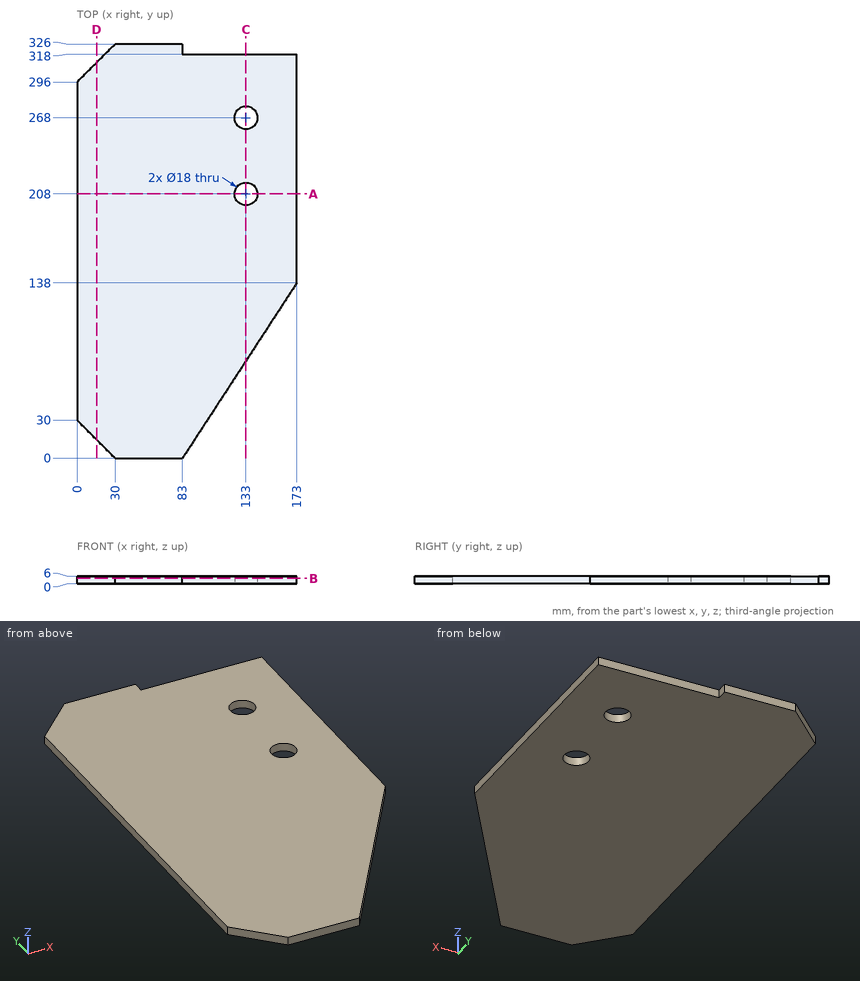
Source: three-view drawing plus pictorial views. Frame: mm from the lowest corner of the part. Coordinates: 2 decimals unless noted, no trailing zeros. Write each loop counter-clockwise with the first axis right and the second up, starting at its lowest first coordinate (ties: lowest second). Pieces come first, ordered by that corner, then holes. Notation, with made-up numbers: (69.5, 43) -> (105.5, 43) arc R25 cw to (105.5, 76) -> close; hole circle Ø1 at (34, 20). An arc over 180 degrees is marked (long way). Answer as a JSON object with one key per item and string values.
1. Section A-A on y = 208. Return the cut outline in (x, z).
Result set:
{"outline": "(0, 0) -> (124, 0) -> (124, 6) -> (0, 6) -> close; (142, 0) -> (173, 0) -> (173, 6) -> (142, 6) -> close"}
2. Section B-B on z = 4.2. Return the cut outline in (x, y).
Result set:
{"outline": "(0, 30) -> (30, 0) -> (83, 0) -> (173, 138) -> (173, 318) -> (83, 318) -> (83, 326) -> (30, 326) -> (0, 296) -> close; hole circle Ø18 at (133, 208); hole circle Ø18 at (133, 268)"}
3. First-contact query: P1, Ø16, axis at x = 133, y = 208, coming from the +Z side; P2, Ø1.8, axis at x = 122, z = 2.5, coming from the +Y side. Flat tips, straight axial feed; report the tip coordinate or a pass-through.
Result set:
{"P1": "passes through", "P2": "stops at y = 318"}
4. Material intervals for line 1 (Y direction, x = 133, z = 2.25); line 2 (X direction, y = 208, z = 2); line 3 (Y direction, x = 138, z = 2), sorted ascending. Write a range as from..to.
Result set:
{"line 1": "y = 76.67..199, 217..259, 277..318", "line 2": "x = 0..124, 142..173", "line 3": "y = 84.33..200.52, 215.48..260.52, 275.48..318"}
5. Section C-C on x = 133. Return the cut outline in (y, z), then the cut area to 3 significant figures.
Result set:
{"outline": "(76.67, 0) -> (199, 0) -> (199, 6) -> (76.67, 6) -> close; (217, 0) -> (259, 0) -> (259, 6) -> (217, 6) -> close; (277, 0) -> (318, 0) -> (318, 6) -> (277, 6) -> close", "area": "1,230 mm2"}
6. Section D-D on x = 15.5. Return the cut outline in (y, z).
Result set:
{"outline": "(14.5, 0) -> (311.5, 0) -> (311.5, 6) -> (14.5, 6) -> close"}
